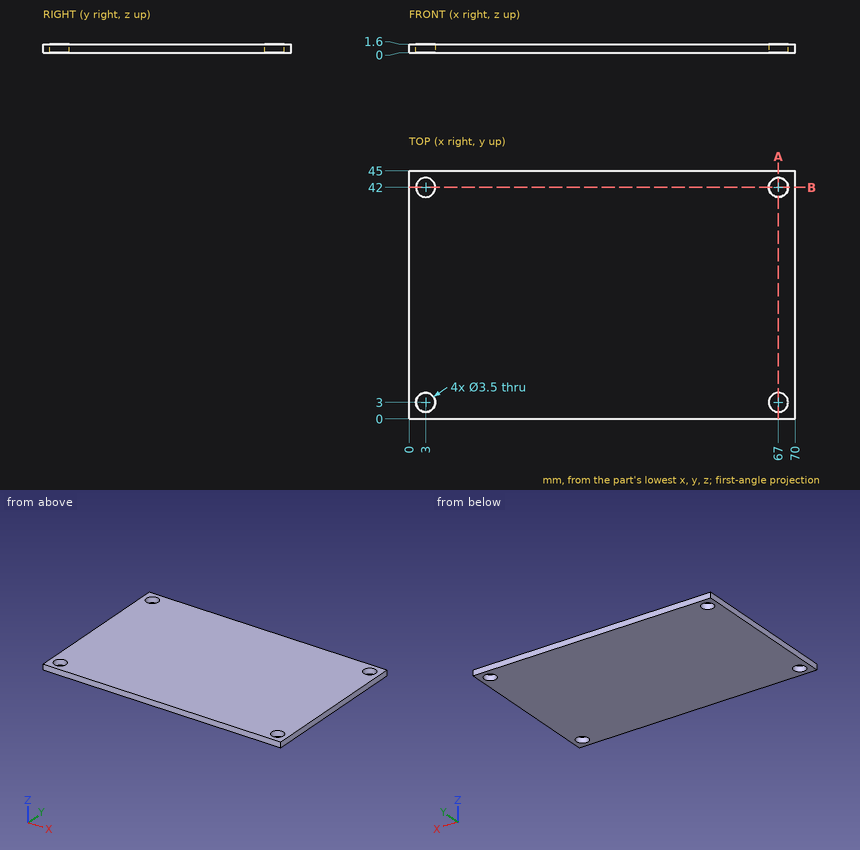
Answer from the drawing. Dimensions are ordinates in mm from the lowest x, y and z of the part. Round coordinates to 2 decimals unless told otherwise and drop trailing zeros. Order: outer loops, then holes, each group sorted by start corner. A loop starts at its lowest first (then second) coordinate and runs counter-clockwise, first axis right, second up. Notation, with made-up numbers: (-30.75, -4.75) - (2.25, -4.75) arc R22 cw to (2.25, 10.25) - close; hole circle Ø4 at (-40, 9). An arc over 180 degrees is marked (long way). Put each result on its own line as item: value. Start each with the question number.
(1) Find section B-B (y = 42). Give the vertices of the cut face in (x, z).
(2) Straight lines are drawn through the part: probe 1 along Y at (x, z) = (3, 1); probe 2 along X at (y, z) = (3, 0.9); probe 3 along X at (y, z) = (4, 0.2). For each, find the intervals that lie inside material, in ascending order. Write a range as from..to.
(3) Find section A-A (x = 67). Give the vertices of the cut face in (y, z).
Reply:
1. outline: (0, 0) - (1.25, 0) - (1.25, 1.6) - (0, 1.6) - close; (4.75, 0) - (65.25, 0) - (65.25, 1.6) - (4.75, 1.6) - close; (68.75, 0) - (70, 0) - (70, 1.6) - (68.75, 1.6) - close
2. probe 1: 0..1.25, 4.75..40.25, 43.75..45
2. probe 2: 0..1.25, 4.75..65.25, 68.75..70
2. probe 3: 0..1.56, 4.44..65.56, 68.44..70
3. outline: (0, 0) - (1.25, 0) - (1.25, 1.6) - (0, 1.6) - close; (4.75, 0) - (40.25, 0) - (40.25, 1.6) - (4.75, 1.6) - close; (43.75, 0) - (45, 0) - (45, 1.6) - (43.75, 1.6) - close
